from build123d import *

# Parameters (mm, degrees)
F1_DEPTH = 12.7
F2_DEPTH = 12.7
F3_R     = 38.1
F4_DEPTH = 25.4
F7_DEPTH = 12.7


with BuildPart() as f1:
    # F0 (on Top) → F1 (new body, symmetric)
    with BuildSketch(Plane.XY):
        with BuildLine():
            Line((0, 152.4), (0, 0))
            Line((0, 0), (203.2, 0))
            ThreePointArc((203.2, 0), (212.1802561211, 3.7197438789), (215.9, 12.7))
            Line((215.9, 12.7), (215.9, 44.45))
            ThreePointArc((215.9, 44.45), (217.7598719395, 48.9401280605), (222.25, 50.8))
            Line((222.25, 50.8), (254, 50.8))
            Line((254, 50.8), (254, 63.5))
            Line((254, 63.5), (215.9, 63.5))
            ThreePointArc((215.9, 63.5), (203.2, 76.2), (215.9, 88.9))
            Line((215.9, 88.9), (254, 88.9))
            Line((254, 88.9), (254, 101.6))
            Line((254, 101.6), (222.25, 101.6))
            ThreePointArc((222.25, 101.6), (217.7598719395, 103.4598719395), (215.9, 107.95))
            Line((215.9, 107.95), (215.9, 139.7))
            ThreePointArc((215.9, 139.7), (212.1802561211, 148.6802561211), (203.2, 152.4))
            Line((203.2, 152.4), (0, 152.4))
        make_face()
        with BuildLine():
            ThreePointArc((101.6, 25.4), (88.9, 38.1), (101.6, 50.8))
            Line((101.6, 50.8), (177.8, 50.8))
            ThreePointArc((177.8, 50.8), (190.5, 38.1), (177.8, 25.4))
            Line((177.8, 25.4), (101.6, 25.4))
        make_face(mode=Mode.SUBTRACT)
        with BuildLine():
            ThreePointArc((101.6, 101.6), (88.9, 114.3), (101.6, 127))
            Line((101.6, 127), (177.8, 127))
            ThreePointArc((177.8, 127), (190.5, 114.3), (177.8, 101.6))
            Line((177.8, 101.6), (101.6, 101.6))
        make_face(mode=Mode.SUBTRACT)
    extrude(amount=F1_DEPTH, both=True)

    # F0 (on Top) → F2 (join)
    with BuildSketch(Plane.XY):
        with BuildLine():
            Line((215.9, 63.5), (254, 63.5))
            Line((254, 63.5), (254, 88.9))
            Line((254, 88.9), (215.9, 88.9))
            ThreePointArc((215.9, 88.9), (203.2, 76.2), (215.9, 63.5))
        make_face()
    extrude(amount=-F2_DEPTH)

    # F3 (on face) → F4 (join)
    with BuildSketch(Plane(origin=(0, 0, 0), x_dir=(0, -1, 0), z_dir=(-1, 0, 0))):
        with BuildLine():
            Line((-152.4, 12.7), (0, 12.7))
            Line((0, 12.7), (0, 114.3))
            ThreePointArc((0, 114.3), (-76.2, 190.5), (-152.4, 114.3))
            Line((-152.4, 114.3), (-152.4, 12.7))
        make_face()
        with Locations((-76.2, 114.3)):
            Circle(F3_R, mode=Mode.SUBTRACT)
    extrude(amount=-F4_DEPTH)

    # F6 (on offset) → F7 (join, symmetric)
    with BuildSketch(Plane.XZ.offset(-76.2)):
        Polygon((63.5, 12.7), (25.4, 63.5), (25.4, 12.7), align=None)
    extrude(amount=F7_DEPTH, both=True)


solid = f1.part
Work out the finished part from the listing and answer in its coordinate system (mm). A direction names the side the tool comes from. Give positions to 0.01 mm unless a question says otherwise; leave off trailing zeros. Order: outer loops, then holes, each group sorted by start corner. A loop starts at its lowest first (then second) coordinate and runs counter-clockwise, first axis right, second up. Notation, with made-up numbers: (72, 42.5) -> (120, 42.5) arc R8 ccw to (120, 46.5) -> close; hole circle Ø4 at (54.5, 85). An arc over 180 degrees is marked (long way). One line per item, written item: value.
Item 1: Flat-ended cylindrical pins translate along their axes: P1, Ø7.5, axis at x = 236, y = 80, coming from the +Z side; P2, Ø20.5, axis at y = 29.5, z = 2.5, coming from the +X side; P3, Ø8, axis at x = 84.5, y = 80.5, coming from the +Z side. Find the tip coordinate at first contact, or state that the pin passes through.
Answer sheet:
P1: z = 0
P2: x = 215.9
P3: z = 12.7
Item 2: Find section C-C, the plane z = 57.5. Give the vertices of the cut face in (x, y), plus the area to 3 significant figures.
Answer sheet:
outline: (0, 0) -> (25.4, 0) -> (25.4, 63.5) -> (29.9, 63.5) -> (29.9, 88.9) -> (25.4, 88.9) -> (25.4, 152.4) -> (0, 152.4) -> close
area: 3,990 mm²
Item 3: Find section B-B, the plane x = 21.5. Give the vertices of the cut face in (y, z), plus the area to 3 significant figures.
Answer sheet:
outline: (0, -12.7) -> (152.4, -12.7) -> (152.4, 114.3) arc R76.2 ccw to (0, 114.3) -> close; hole circle Ø76.2 at (76.2, 114.3)
area: 23,900 mm²
Item 4: A tool of negligible diameter and unlimited length cuts with its end or side. For faces 1 (the flat face through (140, 25.4, 0)), 2 (the flat face through (36, 88.9, 27)), 3 (the flat face through (25.4, 111, 83)), 4 (the flat face through (215.9, 124, 0)), from which of +Z, -Z, +X, -X, +Y, -Y can it reach the whole face along a straight path? Write none if from no direction.
Answer sheet:
face 1: +Z, -Z
face 2: +Z, +X, +Y
face 3: +Z, +X
face 4: +Z, -Z, +X, +Y
Item 5: Determine the mould class of faces 5 (the cylindrical face through (88.903, 37.821, 0.178)), 6 (the cylindrical face through (217.81, 103.41, 0.18)), 7 (the cylindrical face through (88.903, 114.021, 0.178)), 8 (the flat face through (36, 63.5, 27)) for opening direction X: released by +X, released by -X, zero draft, split by the parting line, or undercut.
Answer sheet:
face 5: undercut
face 6: released by +X
face 7: undercut
face 8: zero draft
Item 6: Straight lines are drawn through the part: probe 1 along Y at (x, z) = (103.5, -4); probe 2 along Z at (x, y) = (5, 76); probe 3 along X at (y, z) = (57.5, 62). For each, find the intervals that lie inside material, in ascending order.
Answer sheet:
probe 1: 0 to 25.4, 50.8 to 101.6, 127 to 152.4
probe 2: -12.7 to 76.2, 152.4 to 190.5
probe 3: 0 to 25.4
Item 7: Find section A-A, the plane y = 76.2. Give the vertices of the cut face in (x, z), plus the area to 3 significant figures.
Answer sheet:
outline: (0, -12.7) -> (254, -12.7) -> (254, 0) -> (203.2, 0) -> (203.2, 12.7) -> (63.5, 12.7) -> (25.4, 63.5) -> (25.4, 76.2) -> (0, 76.2) -> close; (0, 152.4) -> (25.4, 152.4) -> (25.4, 190.5) -> (0, 190.5) -> close
area: 9,350 mm²
Item 8: Find section D-D, the plane y = 98. Give the vertices of the cut face in (x, z).
Answer sheet:
outline: (0, -12.7) -> (254, -12.7) -> (254, 12.7) -> (25.4, 12.7) -> (25.4, 83.05) -> (0, 83.05) -> close; (0, 145.55) -> (25.4, 145.55) -> (25.4, 187.32) -> (0, 187.32) -> close
